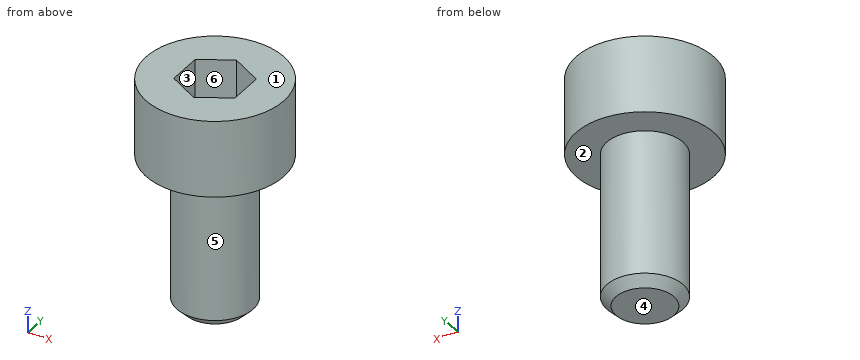
```python
from build123d import *

# Parameters (mm, degrees)
SKETCH1_R           = 2.25
BOSS_EXTRUDE1_DEPTH = 2.5
SKETCH2_R           = 1.25
BOSS_EXTRUDE2_DEPTH = 5
CHAMFER1_SIZE       = 0.3
CUT_EXTRUDE1_DEPTH  = 2


with BuildPart() as part:
    # Sketch1 → Boss-Extrude1 (new body)
    with BuildSketch(Plane.XY):
        Circle(SKETCH1_R)
    extrude(amount=BOSS_EXTRUDE1_DEPTH)

    # Sketch2 → Boss-Extrude2 (add)
    with BuildSketch(Plane(origin=(0, 0, 0), x_dir=(-1, 0, 0), z_dir=(0, 0, -1))):
        Circle(SKETCH2_R)
    extrude(amount=BOSS_EXTRUDE2_DEPTH)

    # Chamfer1
    chamfer1_edges = [part.edges().sort_by_distance(p)[0] for p in [
        (1.25, 0, -5),
    ]]
    chamfer(chamfer1_edges, length=CHAMFER1_SIZE)

    # Sketch3 → Cut-Extrude1 (cut)
    with BuildSketch(Plane.XY.offset(2.5)):
        Polygon((0, 1.154700538), (-1, 0.577350269), (-1, -0.577350269), (0, -1.154700538), (1, -0.577350269), (1, 0.577350269), align=None)
    extrude(amount=-CUT_EXTRUDE1_DEPTH, mode=Mode.SUBTRACT)


solid = part.part
```
Can you work these out from the model? Positions are in its coordinate system, mm. Face numbers are marked on the shaded views. A direction names the side the tool comes from. Round coordinates to 2 decimals unless told otherwise and drop trailing zeros. Loops run counter-clockwise (first coordinate to the right, second up) from the corner with the lowest first, then second, coordinate; pieces in that order, holes last. Notation, with made-up numbers: M -1,37 L 39,37 A19 cw 39,43 Z; hole C 71,76 d1. An arc over 180 degrees is marked long. Answer as a JSON object with one key per item and string values. Group by question number.
Q1. Imagine slicing it at B-B, the plane z = -0.75. Please give me the cut outline in (x, y), then the cut area to 3 significant figures.
Q2. We'd pull the mould along Y, two halves only. Please class the marked faces 3, 4, 5 and 6: +Y half, -Y half, draft (parallel to the pull), parting line (faces both ways), or undercut.
Q3. Imagine slicing it at C-C, the plane x = 1.5. Please give me the cut outline in (y, z).
Q4. Imagine slicing it at D-D, the plane y = -1.8. Please give me the cut outline in (x, z).
Q5. Please list where these lines run through material, in increasing order: L1, parallel to Z at x = 0.2, y = 0.55; L2, parallel to Z at x = -1.4, y = 0.7; L3, parallel to Y at x = 0.9, z = 0.75.
Q6. Will these pins go through, and if not, where does the flat tip stop? pin 1 (2 mm diameter, centred on y = -0.5, z = -2.5, fed in from +X); pin 2 (1 mm diameter, centred on x = 0, y = -0.5, fed in from +Z); pin 3 (1.5 mm diameter, centred on x = 1, z = -2, fed in from +Y).
Q7. On a 3-axis mill with a long thin cutter (end or side, diameter ignored), from which of +Z, -Z, +X, -X, +Y, -Y can I reach the whole of each face in a straight line? I mean the marked faces 1 and 2. Say none if no direction works.
Q8. Imagine slicing it at A-A, the plane y = 0. Please give me the cut outline in (x, z).
Findings:
{
 "1": {"outline": "C 0,0 d2.5", "area": "4.91 mm2"},
 "2": {"face 3": "undercut", "face 4": "draft", "face 5": "parting line", "face 6": "undercut"},
 "3": {"outline": "M -1.68,0 L 1.68,0 L 1.68,2.5 L -1.68,2.5 Z"},
 "4": {"outline": "M -1.35,0 L 1.35,0 L 1.35,2.5 L -1.35,2.5 Z"},
 "5": {"L1": "z = -5 to 0.5", "L2": "z = 0 to 2.5", "L3": "y = -2.06 to -0.64, 0.64 to 2.06"},
 "6": {"pin 1": "stops at x = 1.25", "pin 2": "stops at z = 0.5", "pin 3": "stops at y = 1.22"},
 "7": {"face 1": "+Z, +X, -X, +Y, -Y", "face 2": "-Z"},
 "8": {"outline": "M -2.25,0 L -1.25,0 L -1.25,-4.7 L -0.95,-5 L 0.95,-5 L 1.25,-4.7 L 1.25,0 L 2.25,0 L 2.25,2.5 L 1,2.5 L 1,0.5 L -1,0.5 L -1,2.5 L -2.25,2.5 Z"}
}
